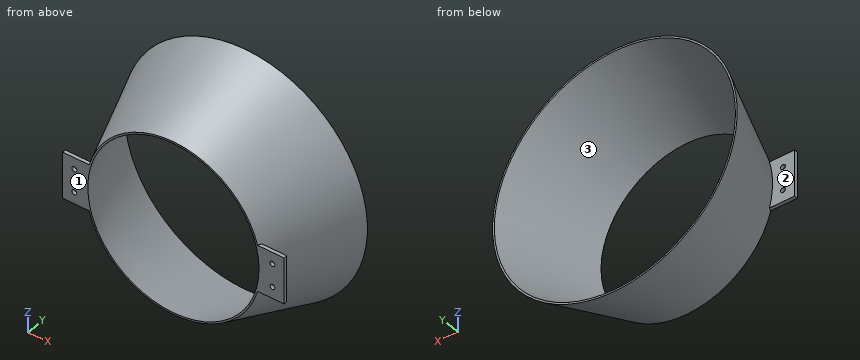
```python
from build123d import *

# Parameters (mm, degrees)
BOSS_EXTRUDE1_DEPTH = 3
SKETCH3_R           = 2.1
CUT_EXTRUDE1_DEPTH  = 3


with BuildPart() as part:
    # Sketch1 → Revolve1 (revolve)
    with BuildSketch(Plane.XY, mode=Mode.PRIVATE) as revolve1_sk:
        Polygon((73.5, 0), (75, 0), (105, 80), (103.5, 80), align=None)
    revolve(revolve1_sk.sketch.rotate(Axis((0, 0, 0), (0, 1, 0)), 90), axis=Axis((0, 0, 0), (0, 1, 0)))

    # Sketch2 → Boss-Extrude1 (add)
    with BuildSketch(Plane.XZ):
        with BuildLine():
            Line((72.284161474, -20), (95, -20))
            Line((95, -20), (95, 20))
            Line((95, 20), (72.284161474, 20))
            ThreePointArc((72.284161474, 20), (75, 0), (72.284161474, -20))
        make_face()
        with BuildLine():
            Line((-95, 20), (-72.284161474, 20))
            ThreePointArc((-72.284161474, 20), (-75, 0), (-72.284161474, -20))
            Line((-72.284161474, -20), (-95, -20))
            Line((-95, -20), (-95, 20))
        make_face()
    extrude(amount=-BOSS_EXTRUDE1_DEPTH)

    # Sketch3 → Cut-Extrude1 (cut)
    with BuildSketch(Plane.XZ):
        with Locations(Location((85, 10, 0), (0, 0, 270))):
            Circle(SKETCH3_R)
        with Locations(Location((85, -10, 0), (0, 0, 90))):
            Circle(SKETCH3_R)
        with Locations(Location((-85, -10, 0), (0, 0, 270))):
            Circle(SKETCH3_R)
        with Locations(Location((-85, 10, 0), (0, 0, 90))):
            Circle(SKETCH3_R)
    extrude(amount=-CUT_EXTRUDE1_DEPTH, mode=Mode.SUBTRACT)


solid = part.part
```
Model file for the job. Use its own axes, mm. Face numbers are marked on the shaded views. Coordinates: 2 decimals unless noted, no trailing zeros. Order: outer loops, then holes, each group sorted by start corner. A loop starts at its lowest first (then second) coordinate and runs counter-clockwise, first axis right, second up. Notation, with made-up numbers: (-22, 54) -> (36, 54) arc R24 ccw to (36, 76) -> close; hole circle Ø10 at (42.5, 6.5). An arc over 180 degrees is marked (long way). Answer as a JSON object with one key per item and string values. Group by question number.
1) Drill centre lines: L1, parallel to X at y = 1.75, z = -10; L2, parallel to X at y = 0.95, z = -10; L3, parallel to X at y = 12.5, z = -34. Where is each one in solid material? Low to high.
2) Cut at C-C, the plane y = 62. Write the cut outline in (x, z), then the cut area to 3 significant figures.
3) Flat gauge pins, fed straight in: pin 1 (0.9 mm diameter, centred on y = 1, z = -1, fed in from -X); pin 2 (1 mm diameter, centred on y = 42, z = -59.5, fed in from +X); pin 3 (6 mm diameter, centred on y = 24.5, z = -33.5, fed in from +X). Where does each tip first touch, or does it go through?
4) Pull direction Y, two halves, no side cores. Call the marked faces 1, 2 and 3: +Y half, -Y half, draft (parallel to the pull), parting line (faces both ways), or undercut.
5) Cut at A-A, the plane z = 0. Write the cut outline in (x, y) (3 decimals).
6) Cut at D-D, the plane y = 21.5. Write the cut outline in (x, z) (1 decimal), then the cut area to 3 significant figures.
7) Cut at B-B, the plane x = 0. Write the cut outline in (y, z).
Check values:
{
 "1": {"L1": "x = -95 to -87.1, -82.9 to -73.48, 73.48 to 82.9, 87.1 to 95", "L2": "x = -95 to -87.1, -82.9 to -73.18, 73.18 to 82.9, 87.1 to 95", "L3": "x = -72.07 to -70.41, 70.41 to 72.07"},
 "2": {"outline": "circle Ø196.5 at (0, 0); hole circle Ø193.5 at (0, 0)", "area": "919 mm²"},
 "3": {"pin 1": "stops at x = -95", "pin 2": "stops at x = 69.02", "pin 3": "stops at x = 78.98"},
 "4": {"face 1": "-Y half", "face 2": "undercut", "face 3": "+Y half"},
 "5": {"outline": "(-105, 80) -> (-76.125, 3) -> (-95, 3) -> (-95, 0) -> (-73.5, 0) -> (-103.5, 80) -> close; (73.5, 0) -> (95, 0) -> (95, 3) -> (76.125, 3) -> (105, 80) -> (103.5, 80) -> close"},
 "6": {"outline": "circle Ø166.1 at (0, 0); hole circle Ø163.1 at (0, 0)", "area": "776 mm²"},
 "7": {"outline": "(0, -75) -> (80, -105) -> (80, -103.5) -> (0, -73.5) -> close; (0, 73.5) -> (80, 103.5) -> (80, 105) -> (0, 75) -> close"}
}
